Check sheet for the modelled part. Datum: model origin and axes. Units: mm. A direction names the side the tool comes from. Round coordinates to 2 decimals unless told otherwise and drop trailing zeros. Write each loop counter-clockwise with the first axis right and the second up, starting at its lowest first coordinate (ties: lowest second). Pieces come first, ordered by that corner, then holes. Notation, with made-up numbers: M 43.25,70.5 L 54.25,70.5 A21 cw 54.25,93.5 Z; hole C 21.25,-15 d7. An arc over 180 degrees is marked long. Answer in a Markdown table with one row per item.
Autodesk Inventor part; units mm, degrees
ref_plane "YZ Plane" through (0, 0, 0) normal (1, 0, 0) x (0, 1, 0)
ref_plane "XZ Plane" through (0, 0, 0) normal (0, 1, 0) x (-1, 0, 0)
ref_plane "XY Plane" through (0, 0, 0) normal (0, 0, 1) x (1, 0, 0)
sketch "Sketch1" plane through (0, 0, 0) normal (0, 0, 1) x (1, 0, 0)
  circle A0 centre (0, 0) radius 50 construction
  line L0 (0, 0) -> (-60, 0)
  circle A1 centre (-60, 0) radius 10
  line L1 (0, 0) -> (-23.6561, 40.9735) construction
  line L2 (0, 0) -> (-50, 0) construction
  line L3 (0, 0) -> (-25, -43.3013)
  line L4 (0, 0) -> (50, 0) construction
  line L5 (0, 0) -> (65, 0) construction
  line L6 (0, 0) -> (30, 51.9615)
  line L7 (0, 0) -> (60, 0) construction
  circle A2 centre (30, 51.9615) radius 10
  arc A3 (35, 60.6218) -> (-70, 0) centre (0, 0) ccw
  arc A4 (25, 43.3013) -> (-50, 0) centre (0, 0) ccw
  line L8 (0, 0) -> (25, 43.3013) construction
  line L9 (0, 0) -> (-50, 0) construction
  line L10 (-60, 0) -> (-63.75, -6.4952)
  line L11 (-60, 0) -> (-52.5, 0) construction
  circle A5 centre (-60, 0) radius 4
  circle A6 centre (-63.75, -6.4952) radius 2.5
  circle A7 centre (0, 0) radius 75 construction
  line L12 (0, 0) -> (-75, 0) construction
  circle A8 centre (-75, 0) radius 5
  line L13 (-25, 43.3013) -> (-35, 60.6218)
  line L14 (0, 0) -> (70, 0) construction
  circle A9 centre (-30, 51.9615) radius 4
  point P0 (25, 43.3013)
  point P1 (-62, -3.4641)
  point P2 (-56, 0)
  dimension "d14" = 20
  dimension "d23" = 150
  dimension "d0" = 100
  dimension "d1" = 60
  dimension "d2" = 20
  dimension "d3" = 60
  dimension "d4" = 120
  dimension "d12" = 60
  dimension "d13" = 60
  dimension "d15" = 120
  dimension "d19" = 7.5
  dimension "d20" = 120
  dimension "d21" = 8
  dimension "d22" = 5
  dimension "d24" = 10
  dimension "d25" = 120
  dimension "d26" = 60
  dimension "d27" = 8
extrude "Extrusion1" add sketch "Sketch1" along normal blind 1 contours A1 A6 L10 A5 L0 | L0 A5 L10 A6 A1 | A1 A3 L13 A9 A4 | A4 L13 A9 A3 A2 | A2 | A6 | A9 L13 | L13 A9
extrude "Extrusion2" add sketch "Sketch1" along normal blind 8 contours A9 L13 | L13 A9
1. Section check B-B, the plane x = -30. Record the cut outline in (y, z).
Found:
| item | result |
|---|---|
| outline | M 40,0 L 63.25,0 L 63.25,1 L 55.96,1 L 55.96,8 L 47.96,8 L 47.96,1 L 40,1 Z |
2. Section check D-D, the plane z = 5.25. Record the cut outline in (x, y).
Found:
| item | result |
|---|---|
| outline | C -30,51.96 d8 |
3. Draft check along X on faces 1 (the face through (-59.8, -10, 0.5)), 2 (the face through (-25.63, 42.93, 0.49)), 3 (the face through (-56.185, -1.201, 0.493)), 4 (the face through (-30, 52, 8)). Enter one of: +X half, -X half, draft (parallel to the pull), parting line (faces both ways), or undercut.
Found:
| item | result |
|---|---|
| face 1 | parting line |
| face 2 | undercut |
| face 3 | undercut |
| face 4 | draft |
4. Section check A-A, the plane x = -60. Record the cut outline in (y, z), and give its area (3 significant figures).
Found:
| item | result |
|---|---|
| outline | M -10,0 L -4,0 L -4,1 L -10,1 Z; M 4,0 L 36.06,0 L 36.06,1 L 4,1 Z |
| area | 38.1 mm2 |
5. Section check C-C, the plane y = 25. Record the cut outline in (x, z).
Found:
| item | result |
|---|---|
| outline | M -65.38,0 L -43.3,0 L -43.3,1 L -65.38,1 Z |
6. Scan lines: L1, parallel to X at y = 0, z = 0.45; L2, parallel to Z at x = -40.5, y = 51.5; L3, parallel to X at y = 51.5, z = 4.75. Record each from-to range of solid material in increasing order.
Found:
| item | result |
|---|---|
| L1 | x = -70 to -64, -56 to -50 |
| L2 | z = 0 to 1 |
| L3 | x = -33.97 to -26.03 |
7. Access from +Z, -Z, +X, -X, +Y, -Y to the whole of each face (thin tool, end or side, straight path). Record for faces 5 (the face through (-35.885, 60.102, 0.493)), 6 (the face through (-30.521, 47.996, 4.451)).
Found:
| item | result |
|---|---|
| face 5 | +Z, -Z, +Y |
| face 6 | +Z |
8. Go/stop test with flat-tipped pins: pin 1 (8 mm diameter, centred on x = -41, y = 39, fed in from +Z); pin 2 (1.5 mm diameter, centred on x = -34, z = 6, fed in from -Y). Record where each tip stops, or that it passes through.
Found:
| item | result |
|---|---|
| pin 1 | stops at z = 1 |
| pin 2 | stops at y = 49.63 |
